Autodesk Inventor part; units mm, degrees
ref_plane "YZ Plane" through (0, 0, 0) normal (1, 0, 0) x (0, 1, 0)
ref_plane "XZ Plane" through (0, 0, 0) normal (0, 1, 0) x (-1, 0, 0)
ref_plane "XY Plane" through (0, 0, 0) normal (0, 0, 1) x (1, 0, 0)
sketch "Sketch1" plane through (0, 0, 0) normal (0, 1, 0) x (-1, 0, 0)
  circle A0 centre (0, 0) radius 600
  circle A1 centre (0, 0) radius 604
  dimension "d0" = 1200
  dimension "d1" = 1208
extrude "Extrusion1" add sketch "Sketch1" along normal blind 100
sketch "Sketch2" plane through (0, 0, 0) normal (0, -1, 0) x (1, 0, 0)
  line L0 (-737.5363, 12.1167) -> (-600.0118, 8.1785)
  line L1 (-256.3877, -691.6444) -> (-210.1448, -562.0678)
  circle A0 centre (0, 0) radius 600
  line L2 (-210.1221, -562.0042) -> (-211.4667, -565.7719)
  circle A1 centre (0, 0) radius 604
  line L3 (-599.9441, 8.1765) -> (-603.943, 8.2911)
  point P0 (-599.9443, 8.1765)
  point P1 (-603.9431, 8.2911)
extrude "Extrusion2" cut sketch "Sketch2" against normal blind 100 contours L0 L3 A0 L2 L1 A1 picked at (-484.3692, -358.2492)
properties part number "Edge Band - Platform A Outer" material "Wood (Birch)"
Input: part model. Units: mm. Frame: model coordinates. Round coordinates to 2 decimals unless told otherwise and drop trailing zeros. Order: outer loops, then holes, each group sorted by start corner. A loop starts at its lowest first (then second) coordinate and runs counter-clockwise, first axis right, second up. Notation, with made-up numbers: (2.5, -26) - (27.5, -26) arc R23 cw to (27.5, 11) - close; hole circle Ø1 at (-7, 9). An arc over 180 degrees is marked (long way). Answer as a JSON object with one key per item and string values. Group by question number.
(1) Material intervals for probe 1 along Z at (x, y) = (0, 64); probe 2 along X at (y, z) = (27.5, 0); probe 3 along Z at (x, y) = (-128, 46), sorted ascending. Write a range as from..to.
(2) Cut plane D-D (z = -137). Return loops of the section in (x, y).
(3) Draft query along Z for faces 1 (the face through (506.98, 49.3, 320.89)), 2 (the face through (510.36, 49.3, 323.03)). Return one class per face: released by +Z, released by -Z, zero draft, split by the parting line, or undercut.
(4) Cut plane C-C (y = 41). Return loops of the section in (x, z).
(5) Pin query (flat end, axial travel): P1, Ø2, axis at x = 322.5, y = 72.5, coming from the +Z side; P2, Ø12, axis at x = 217, y = 50, coming from the -Z side; P3, Ø3, axis at y = 14.5, z = -154.5, coming from the +X side. Return the tip coordinate at first contact, or that it passes through.
(6) Cut plane A-A (x = 0). Return loops of the section in (y, z).
(7) Cut plane B-B (z = 384). Return loops of the section in (x, y).
Here are the results:
{
 "1": {"probe 1": "z = -604..-600, 600..604", "probe 2": "x = 600..604", "probe 3": "z = -590.28..-586.19, 586.19..590.28"},
 "2": {"outline": "(584.15, 0) - (588.26, 0) - (588.26, 100) - (584.15, 100) - close"},
 "3": {"face 1": "undercut", "face 2": "split by the parting line"},
 "4": {"outline": "(-603.94, 8.29) - (-600.01, 8.18) - (-599.94, 8.18) arc R600 cw (long way) to (-210.12, -562) - (-210.14, -562.07) - (-211.47, -565.77) arc R604 ccw (long way) to start"},
 "5": {"P1": "stops at z = 511.33", "P2": "stops at z = -565.95", "P3": "stops at x = 584.3"},
 "6": {"outline": "(0, -604) - (100, -604) - (100, -600) - (0, -600) - close; (0, 600) - (100, 600) - (100, 604) - (0, 604) - close"},
 "7": {"outline": "(-466.22, 0) - (-461.02, 0) - (-461.02, 100) - (-466.22, 100) - close; (461.02, 0) - (466.22, 0) - (466.22, 100) - (461.02, 100) - close"}
}
